Design review of the part built by this model. Coordinates are the model's own, in mm. Face numbers are marked on the shaded views. A direction names the side the tool comes from. Coordinates: 2 decimals unless noted, no trailing zeros. Loops run counter-clockwise (first coordinate to the right, second up) from the corner with the lowest first, then second, coordinate; pieces in that order, holes last.
Autodesk Inventor part; units mm, degrees
ref_plane "YZ Plane" through (0, 0, 0) normal (1, 0, 0) x (0, 1, 0)
ref_plane "XZ Plane" through (0, 0, 0) normal (0, 1, 0) x (-1, 0, 0)
ref_plane "XY Plane" through (0, 0, 0) normal (0, 0, 1) x (1, 0, 0)
sketch "Sketch1" plane through (0, 0, 0) normal (0, 0, 1) x (1, 0, 0)
  circle A0 centre (0, 0) radius 11.1125
  circle A1 centre (0, 0) radius 57.15 construction
  line L0 (29.571, 44.45) -> (35.921, 44.45) construction
  line L1 (35.921, 44.45) -> (35.921, -44.45) construction
  line L2 (35.921, -44.45) -> (29.571, -44.45) construction
  line L3 (29.571, -44.45) -> (29.571, 44.45) construction
  line L4 (31.75, 47.519) -> (31.75, -47.519)
  arc A2 (31.75, 47.519) -> (31.75, -47.519) centre (0, 0) ccw
  point P0 (29.571, 0)
  point P1 (57.15, 0)
  point P2 (35.921, 0)
  dimension "d0" = 22.225
  dimension "d2" = 114.3
  dimension "d3" = 88.9
  dimension "d4" = 6.35
  dimension "d5" = 35.921
  dimension "d6" = 21.229
  dimension "d7" = 31.75
extrude "Extrusion1" add sketch "Sketch1" along normal mid plane 82.55
sketch "Sketch3" plane through (0, 0, 41.275) normal (0, 0, 1) x (1, 0, 0)
  circle A0 centre (0, 0) radius 11.1125 construction
  arc A1 (31.75, 47.519) -> (31.75, -47.519) centre (0, 0) ccw construction
  line L0 (31.75, 47.519) -> (31.75, -47.519) construction
  circle A2 centre (0, 0) radius 11.1125 construction
  circle A3 centre (0, 0) radius 23.8125
  dimension "d10" = 47.625
extrude "Extrusion2" cut sketch "Sketch3" against normal blind 12.7
sketch "Sketch4" plane through (0, 0, -41.275) normal (0, 0, -1) x (-1, 0, 0)
  circle A0 centre (0, 0) radius 23.8125
  dimension "d13" = 47.625
extrude "Extrusion3" cut sketch "Sketch4" against normal blind 12.7
sketch "Sketch7" plane through (31.75, -47.519, 41.275) normal (1, 0, 0) x (0, 0, -1)
  line L0 (28.575, 22.119) -> (53.975, 22.119) construction
  line L1 (53.975, 22.119) -> (53.975, 72.919) construction
  line L2 (53.975, 72.919) -> (28.575, 72.919) construction
  line L3 (28.575, 72.919) -> (28.575, 22.119) construction
  line L4 (28.575, 22.119) -> (53.975, 72.919) construction
  line L5 (53.975, 22.119) -> (28.575, 72.919) construction
  line L6 (31.75, 25.294) -> (50.8, 25.294) construction
  line L7 (50.8, 25.294) -> (50.8, 69.744) construction
  line L8 (50.8, 69.744) -> (31.75, 69.744) construction
  line L9 (31.75, 69.744) -> (31.75, 25.294) construction
  line L10 (31.75, 25.294) -> (50.8, 69.744) construction
  line L11 (50.8, 25.294) -> (31.75, 69.744) construction
  line L12 (50.673, 25.421) -> (31.877, 25.421)
  line L13 (31.877, 25.421) -> (31.877, 69.617)
  line L14 (31.877, 69.617) -> (50.673, 69.617)
  line L15 (50.673, 69.617) -> (50.673, 25.421)
  line L16 (50.673, 25.421) -> (31.877, 69.617) construction
  line L17 (31.877, 25.421) -> (50.673, 69.617) construction
  point P0 (41.275, 47.519)
  dimension "d34" = 25.4
  dimension "d35" = 50.8
  dimension "d36" = 3.175
  dimension "d37" = 3.175
  dimension "d38" = 0.127
  dimension "d39" = 0.127
extrude "Extrusion5" add sketch "Sketch7" along normal blind 25.4
sketch "Sketch8" plane through (0, 0, 0) normal (0, 0, 1) x (1, 0, 0)
  circle A0 centre (0, 0) radius 11.1125
  arc A1 (31.75, 47.519) -> (31.75, -47.519) centre (0, 0) ccw
  line L0 (31.75, 47.519) -> (31.75, 22.098)
  line L1 (31.75, 22.098) -> (57.15, 22.098)
  line L2 (57.15, 22.098) -> (57.15, -22.098)
  line L3 (57.15, -22.098) -> (31.75, -22.098)
  line L4 (31.75, -22.098) -> (31.75, -47.519)
  arc A2 (31.75, 47.519) -> (31.75, -47.519) centre (0, 0) ccw
  line L5 (12.7, 55.721) -> (12.7, -55.721)
  dimension "d42" = 12.7
extrude "Extrusion6" cut sketch "Sketch8" along normal mid plane 50.8 contours L5 A1
sketch "Sketch9" plane through (31.75, -22.098, 9.398) normal (0, 0, 1) x (1, 0, 0)
  line L0 (25.4, 44.196) -> (25.4, 0)
  point P0 (-31.75, 22.098)
  point P1 (12.7, 34.798)
  point P2 (12.7, 22.098)
  point P3 (12.7, 9.398)
  point P4 (25.4, 22.098)
  dimension "d45" = 12.7
  dimension "d46" = 12.7
  dimension "d47" = 12.7
hole "Hole2" at (44.45, 12.7, 9.398) at (44.45, 0, 9.398) at (44.45, -12.7, 9.398) direction (0, 0, -1) diameter 3.9624 end through all
fillet "Fillet1" radius 1.27 8 edges at (57.15, 0, 9.398) (57.15, 22.098, 0) (57.15, 0, -9.398) (57.15, -22.098, 0) (44.45, -22.098, 9.398) (44.45, 22.098, 9.398) (44.45, 22.098, -9.398) (44.45, -22.098, -9.398)
equation "\"d13\" = d10"
equation "\"d14\" = d11"
equation "\"d37\" = d36"
equation "\"d39\" = d38"
properties part number "EL2-A-008" material "Aluminum 6061"
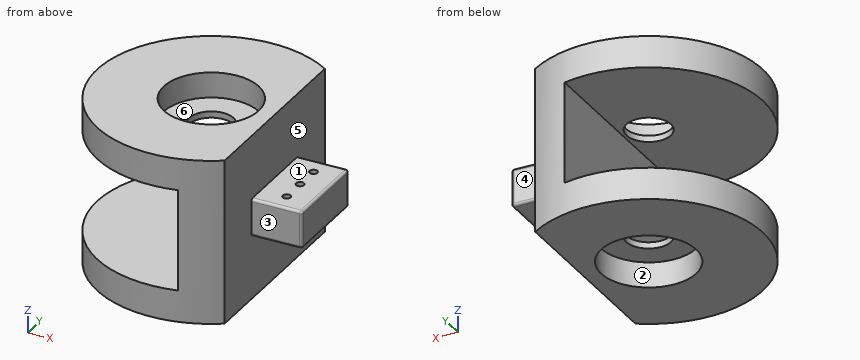
Q1. Take a section at B-B, the plane x = 44.45. Write out the cut boundary in (y, z).
Q2. Machinability: for the marked faces 1, 2 and 3, which of the approach directions +Z, -Z, +X, -X, +Y, -Y give a long, thin tool a straight path to every point of the face, cutting with its end or side? Answer none if there is none.
Q3. For line 1 (Y direction, x = 44.45, z = 3.5); line 2 (Z direction, x = 7.5, y = -45.5) (3 decimals); line 3 (Z direction, x = -3, y = -22.5) (3 decimals), list the stretches that pass through material, from the lowest coordinate up.
Q4. Clearance check with flat-ended pins moving along their axes: pin 1 Ø6.5 at (x, y) = (44.45, 12.7) entering from -Z; pin 2 Ø18 at (x, z) = (44, -2.5) entering from +Y; pin 3 Ø8 at (x, z) = (-29.5, -25) entering from +Y; pin 4 Ø20 at (x, y) = (0, 0) entering from +Z. State where each tip first meets the part, or that it passes through.
Q5. Take a section at A-A, the plane y = 0. Give the number of separate pieces and of enclosed holes in the cut face, then the cut area to 3 significant figures.
Q6. Take a section at D-D, the plane y = -18. Write out the cut boundary in (x, z) (3 decimals), then the cut area to 3 significant figures.
Q7. The part is to be moulded in two halves that separate along X. For the marked faces 4, 5 and 6, say which applies: pulls with the +X half, pulls with the -X half, needs draft (parallel to the pull), parting line crosses it, or undercut.
Q8. Take a section at C-C, the plane z = 4. Write out the cut boundary in (x, y), then the cut area to 3 significant figures.
Entries:
1. outline: (-22.1, -8.13) arc R1.27 ccw to (-20.83, -9.4) - (-14.68, -9.4) - (-14.68, 9.4) - (-20.83, 9.4) arc R1.27 ccw to (-22.1, 8.13) - close; (-10.72, -9.4) - (-1.98, -9.4) - (-1.98, 9.4) - (-10.72, 9.4) - close; (1.98, -9.4) - (10.72, -9.4) - (10.72, 9.4) - (1.98, 9.4) - close; (14.68, -9.4) - (20.83, -9.4) arc R1.27 ccw to (22.1, -8.13) - (22.1, 8.13) arc R1.27 ccw to (20.83, 9.4) - (14.68, 9.4) - close
2. face 1: +Z, +X, +Y, -Y
2. face 2: -Z
2. face 3: +Z, -Z, +X, -Y
3. line 1: y = -22.1 to -14.68, -10.72 to -1.98, 1.98 to 10.72, 14.68 to 22.1
3. line 2: z = -41.275 to -25.4, 25.4 to 41.275
3. line 3: z = -28.575 to -25.4, 25.4 to 28.575
4. pin 1: stops at z = -9.4
4. pin 2: stops at y = 22.1
4. pin 3: stops at y = 51.14
4. pin 4: passes through
5. separate pieces: 4
5. enclosed holes: 0
5. area: 2,840 mm2
6. outline: (-54.241, -41.275) - (-15.59, -41.275) - (-15.59, -28.575) - (15.59, -28.575) - (15.59, -41.275) - (31.75, -41.275) - (31.75, -9.398) - (55.88, -9.398) arc R1.27 ccw to (57.15, -8.128) - (57.15, 8.128) arc R1.27 ccw to (55.88, 9.398) - (31.75, 9.398) - (31.75, 41.275) - (15.59, 41.275) - (15.59, 28.575) - (-15.59, 28.575) - (-15.59, 41.275) - (-54.241, 41.275) - (-54.241, 25.4) - (12.7, 25.4) - (12.7, -25.4) - (-54.241, -25.4) - close
6. area: 3,380 mm2
7. face 4: needs draft
7. face 5: pulls with the +X half
7. face 6: undercut
8. outline: (12.7, -55.72) arc R57.15 ccw to (31.75, -47.52) - (31.75, -22.1) - (55.88, -22.1) arc R1.27 ccw to (57.15, -20.83) - (57.15, 20.83) arc R1.27 ccw to (55.88, 22.1) - (31.75, 22.1) - (31.75, 47.52) arc R57.15 ccw to (12.7, 55.72) - close; hole circle Ø3.96 at (44.45, -12.7); hole circle Ø3.96 at (44.45, 0); hole circle Ø3.96 at (44.45, 12.7)
8. area: 3,080 mm2
